Could you check a few things on this model? Use its own coordinates, in mm. A direction names the side the tool comes from. Round coordinates to 2 decimals unless told otherwise and drop trailing zeros. Loops run counter-clockwise (first coordinate to the right, second up) from the corner with the lowest first, then second, coordinate; pieces in that order, holes last. Notation, with made-up numbers: (24, 30) -> (75, 30) arc R25 ccw to (75, 56) -> close; hole circle Ø4 at (-12, 3). An arc over 180 degrees is marked (long way). One line per item, written item: value.
from build123d import *

# Parameters (mm, degrees)
BOSS_EXTRUDE1_DEPTH   = 5
SKETCH2_W             = 20
SKETCH2_H             = 40
SKETCH2_W_2           = 5
SKETCH2_H_2           = 20
BOSS_EXTRUDE2_DEPTH   = 20
SKETCH3_W             = 48.5
SKETCH3_H             = 25
BOSS_EXTRUDE3_DEPTH   = 4
SKETCH4_W             = 48.5
SKETCH4_H             = 25
BOSS_EXTRUDE4_DEPTH   = 4
SKETCH6_W             = 293.991294913
SKETCH6_H             = 166.612051016
CUT_EXTRUDE1_DEPTH    = 218
SKETCH7_W             = 4
SKETCH7_H             = 48
BOSS_EXTRUDE5_DEPTH   = 20
SKETCH8_W             = 48
SKETCH8_H             = 1
CUT_EXTRUDE2_DEPTH    = 87
SKETCH9_R             = 1
CUT_EXTRUDE3_DEPTH    = 10
SKETCH10_R            = 1
CUT_EXTRUDE4_DEPTH    = 60
SKETCH12_R            = 3
CUT_EXTRUDE5_DEPTH    = 29.5
SKETCH13_R            = 1
CUT_EXTRUDE6_DEPTH    = 29.5
SKETCH14_R            = 1
CUT_EXTRUDE7_DEPTH    = 29.5
SKETCH15_R            = 1.775
CUT_EXTRUDE8_DEPTH    = 29.5
SKETCH16_R            = 2.025
CUT_EXTRUDE9_DEPTH    = 29.5
SKETCH17_R            = 3.5
CUT_EXTRUDE10_DEPTH   = 3
SKETCH18_W            = 48
SKETCH18_H            = 44
SKETCH18_R            = 2.025
SKETCH18_R_2          = 3
BOSS_EXTRUDE6_DEPTH   = 2
CROQUIS2_R            = 4
CORTAR_EXTRUIR2_DEPTH = 0.5


with BuildPart() as part:
    # Sketch1 → Boss-Extrude1 (new body)
    with BuildSketch(Plane(origin=(0, 0, 0), x_dir=(1, 0, 0), z_dir=(0, 1, 0))):
        Polygon((-5, 20), (43.5, 20), (43.5, 35), (73.5, 35), (73.5, -15), (43.5, -15), (43.5, 0), (-5, 0), align=None)
    extrude(amount=BOSS_EXTRUDE1_DEPTH)

    # Sketch2 → Boss-Extrude2 (add)
    with BuildSketch(Plane(origin=(0, 5, 0), x_dir=(1, 0, 0), z_dir=(0, 1, 0))):
        Polygon((40, 20), (43.5, 20), (43.5, 35), (73.5, 35), (73.5, -15), (43.5, -15), (43.5, 0), (40, 0), align=None)
        with Locations((58.5, 10)):
            Rectangle(SKETCH2_W, SKETCH2_H, mode=Mode.SUBTRACT)
        with Locations((-2.5, 10)):
            Rectangle(SKETCH2_W_2, SKETCH2_H_2)
    extrude(amount=BOSS_EXTRUDE2_DEPTH)

    # Sketch3 → Boss-Extrude3 (add)
    with BuildSketch(Plane.XY):
        with Locations((19.25, 12.5)):
            Rectangle(SKETCH3_W, SKETCH3_H)
    extrude(amount=BOSS_EXTRUDE3_DEPTH)

    # Sketch4 → Boss-Extrude4 (add)
    with BuildSketch(Plane(origin=(0, 0, -20), x_dir=(-1, 0, 0), z_dir=(0, 0, -1))):
        with Locations((-19.25, 12.5)):
            Rectangle(SKETCH4_W, SKETCH4_H)
    extrude(amount=BOSS_EXTRUDE4_DEPTH)

    # Sketch6 → Cut-Extrude1 (cut)
    with BuildSketch(Plane.XZ):
        with Locations((19.737100805, -5.654680936)):
            Rectangle(SKETCH6_W, SKETCH6_H)
        Polygon((72.5, -34), (72.5, 14), (44.5, 14), (44.5, 4), (43.5, 4), (42.175115589, 8.832020086), (-3.564522491, 8.832020086), (-4, 4), (-4, -32.651206012), (43.5, -34), align=None, mode=Mode.SUBTRACT)
    extrude(amount=-CUT_EXTRUDE1_DEPTH, mode=Mode.SUBTRACT)

    # Sketch7 → Boss-Extrude5 (add)
    with BuildSketch(Plane(origin=(0, 25, 0), x_dir=(1, 0, 0), z_dir=(0, 1, 0))):
        with Locations((70.5, 10)):
            Rectangle(SKETCH7_W, SKETCH7_H)
    extrude(amount=BOSS_EXTRUDE5_DEPTH)

    # Sketch8 → Cut-Extrude2 (cut)
    with BuildSketch(Plane.ZY.offset(4)):
        with Locations((-10, 0.5)):
            Rectangle(SKETCH8_W, SKETCH8_H)
    extrude(amount=-CUT_EXTRUDE2_DEPTH, mode=Mode.SUBTRACT)

    # Sketch9 → Cut-Extrude3 (cut)
    with BuildSketch(Plane.ZY.offset(4)):
        with Locations((-2.5, 22.5)):
            Circle(SKETCH9_R)
        with Locations((-17.5, 22.5)):
            Circle(SKETCH9_R)
        with Locations((-17.5, 7.5)):
            Circle(SKETCH9_R)
        with Locations((-2.5, 7.5)):
            Circle(SKETCH9_R)
    extrude(amount=-CUT_EXTRUDE3_DEPTH, mode=Mode.SUBTRACT)

    # Sketch10 → Cut-Extrude4 (cut)
    with BuildSketch(Plane.ZY.offset(-40)):
        with Locations((-3, 15)):
            Circle(SKETCH10_R)
        with Locations((-10, 8)):
            Circle(SKETCH10_R)
        with Locations((-17, 15)):
            Circle(SKETCH10_R)
    extrude(amount=-CUT_EXTRUDE4_DEPTH, mode=Mode.SUBTRACT)

    # Sketch12 → Cut-Extrude5 (cut)
    with BuildSketch(Plane(origin=(72.5, 0, 0), x_dir=(0, 0, -1), z_dir=(1, 0, 0))):
        with Locations((17, 15)):
            Circle(SKETCH12_R)
        with Locations((10, 8)):
            Circle(SKETCH12_R)
        with Locations((3, 15)):
            Circle(SKETCH12_R)
    extrude(amount=-CUT_EXTRUDE5_DEPTH, mode=Mode.SUBTRACT)

    # Sketch13 → Cut-Extrude6 (cut)
    with BuildSketch(Plane.XY.offset(14)):
        with Locations((58.5, 8)):
            Circle(SKETCH13_R)
        with Locations((51.5, 15)):
            Circle(SKETCH13_R)
        with Locations((65.5, 15)):
            Circle(SKETCH13_R)
    extrude(amount=-CUT_EXTRUDE6_DEPTH, mode=Mode.SUBTRACT)

    # Sketch14 → Cut-Extrude7 (cut)
    with BuildSketch(Plane.XY.offset(-30)):
        with Locations((66, 22.5)):
            Circle(SKETCH14_R)
        with Locations((66, 7.5)):
            Circle(SKETCH14_R)
        with Locations((51, 7.5)):
            Circle(SKETCH14_R)
        with Locations((51, 22.5)):
            Circle(SKETCH14_R)
    extrude(amount=-CUT_EXTRUDE7_DEPTH, mode=Mode.SUBTRACT)

    # Sketch15 → Cut-Extrude8 (cut)
    with BuildSketch(Plane(origin=(72.5, 0, 0), x_dir=(0, 0, -1), z_dir=(1, 0, 0))):
        with Locations((10, 35)):
            Circle(SKETCH15_R)
    extrude(amount=-CUT_EXTRUDE8_DEPTH, mode=Mode.SUBTRACT)

    # Sketch16 → Cut-Extrude9 (cut)
    with BuildSketch(Plane.ZY.offset(-68.5)):
        with Locations((-10, 35)):
            Circle(SKETCH16_R)
    extrude(amount=-CUT_EXTRUDE9_DEPTH, mode=Mode.SUBTRACT)

    # Sketch17 → Cut-Extrude10 (cut)
    with BuildSketch(Plane.ZY.offset(-68.5)):
        with Locations((-10, 35)):
            Circle(SKETCH17_R)
    extrude(amount=-CUT_EXTRUDE10_DEPTH, mode=Mode.SUBTRACT)

    # Sketch18 → Boss-Extrude6 (add)
    with BuildSketch(Plane(origin=(72.5, 0, 0), x_dir=(0, 0, -1), z_dir=(1, 0, 0))):
        with Locations((10, 23)):
            Rectangle(SKETCH18_W, SKETCH18_H)
        with Locations((10, 35)):
            Circle(SKETCH18_R, mode=Mode.SUBTRACT)
        with Locations((17, 15)):
            Circle(SKETCH18_R_2, mode=Mode.SUBTRACT)
        with Locations((10, 8)):
            Circle(SKETCH18_R_2, mode=Mode.SUBTRACT)
        with Locations((3, 15)):
            Circle(SKETCH18_R_2, mode=Mode.SUBTRACT)
    extrude(amount=BOSS_EXTRUDE6_DEPTH)

    # Croquis2 → Cortar-Extruir2 (cut)
    with BuildSketch(Plane(origin=(74.5, 0, 0), x_dir=(0, 0, -1), z_dir=(1, 0, 0))):
        with Locations((10, 35)):
            Circle(CROQUIS2_R)
    extrude(amount=-CORTAR_EXTRUIR2_DEPTH, mode=Mode.SUBTRACT)


solid = part.part
(1) I'm going to push flat-ended pins straight in: pin 1 Ø5.5 at (y, z) = (35, -10) entering from +X; pin 2 Ø1.2 at (x, y) = (66, 22.5) entering from -Z; pin 3 Ø1.5 at (x, y) = (15.5, 14.5) entering from -Z. Where does each tip first touch, or does it pass through?
Recorded:
pin 1: x = 74
pin 2: z = 10
pin 3: z = -24
(2) If we section it at B-B, the plane y = 22.5: Give the number of separate pieces and of enclosed holes in the cut face, then the cut area to 3 significant figures.
Recorded:
separate pieces: 3
enclosed holes: 0
area: 1,180 mm²
(3) If we section it at C-C, the plane z = 3: Please give me the cut outline in (x, y), then the cut area to 3 significant figures.
Recorded:
outline: (-4, 1) -> (74.5, 1) -> (74.5, 45) -> (68.5, 45) -> (68.5, 5) -> (48.5, 5) -> (48.5, 25) -> (-4, 25) -> close
area: 1,600 mm²
(4) For faces 1 (the face through (20, 13, -24)), 2 (the face through (45.79, 12.07, -2.35)), 3 (the face through (40, 15, -10)), 4 (the face through (-2.03, 8.49, -2.63)), 5 (the face through (44.5, 13, 9)), which set-ups out of +Z, -Z, +X, -X, +Y, -Y let a thin tool reach every point of the face, with its end or its side?
Recorded:
face 1: -Z, -X, +Y, -Y
face 2: +X
face 3: +Y
face 4: -X
face 5: +Z, -X, +Y, -Y
(5) If we section it at A-A, the plane x = 58.5: Please give me the cut outline in (y, z).
Recorded:
outline: (1, -34) -> (25, -34) -> (25, -30) -> (5, -30) -> (5, 10) -> (7, 10) -> (7, 14) -> (1, 14) -> close; (9, 10) -> (25, 10) -> (25, 14) -> (9, 14) -> close
(6) If we section it at D-D, the plane x = 8: Please give me the cut outline in (y, z), then the cut area to 3 significant figures.
Recorded:
outline: (1, -24) -> (25, -24) -> (25, -20) -> (5, -20) -> (5, 0) -> (25, 0) -> (25, 4) -> (1, 4) -> close
area: 272 mm²
(7) If I drill on L1, parallel to X at y = 13.5, z = -14; L2, parallel to Y at x = 73.45, z = -3; L3, parallel to Z at x = 13.5, y = 11, over which ranges is the centre line in solid material (lowest first)?
Recorded:
L1: -4 to 0, 40 to 48.5, 68.5 to 74.5
L2: 1 to 12, 18 to 45
L3: -24 to -20, 0 to 4
(8) Thinking about a two-plate mould opening in X: for faces 6 (the face through (51.96, 14.11, 12.03)), 7 (the face through (43, 16, -16)), 8 (the face through (20, 5, -10)), 9 (the face through (-2.028, 7.8, -16.546)), which applies, released by +X, released by -X, zero draft, split by the parting line, or undercut?
Recorded:
face 6: undercut
face 7: released by +X
face 8: undercut
face 9: zero draft
